Input: part model. Units: mm. Frame: model coordinates. A direction names the side the tool comes from. Coordinates: 2 decimals unless noted, no trailing zeros. Order: outer loops, then holes, each group sorted by start corner. A loop starts at its lowest first (then second) coordinate and runs counter-clockwise, first axis right, second up.
from build123d import *

# Parameters (mm, degrees)
F1_W     = 2334
F1_H     = 613
F2_DEPTH = 29
F4_DEPTH = 871
F3_W     = 45
F3_H     = 463
F3_W_2   = 392
F3_H_2   = 45
F3_W_3   = 525
F7_DEPTH = 95
F3_W_4   = 70
F8_DEPTH = 750
F6_W     = 2184
F6_H     = 553
F6_W_2   = 45
F6_H_2   = 463
F9_DEPTH = 95


with BuildPart() as f2:
    # F1 (on offset) → F2 (new body)
    with BuildSketch(Plane.XY.offset(900)):
        Rectangle(F1_W, F1_H)
    extrude(amount=-F2_DEPTH)

    # F3 (on face) → F4 (join)
    with BuildSketch(Plane(origin=(0, 0, 871), x_dir=(1, 0, 0), z_dir=(0, 0, -1))):
        Polygon((-1022, 256.5), (-1117, 256.5), (-1117, 211.5), (-1072, 211.5), (-1022, 211.5), align=None)
        Polygon((-1072, -251.5), (-1117, -251.5), (-1117, -296.5), (-1022, -296.5), (-1022, -251.5), align=None)
        Polygon((1117, -296.5), (1117, -251.5), (1072, -251.5), (1022, -251.5), (1022, -296.5), align=None)
        Polygon((1117, 256.5), (1022, 256.5), (1022, 211.5), (1072, 211.5), (1117, 211.5), align=None)
        Polygon((35, 256.5), (-35, 256.5), (-35, 211.5), (-22.5, 211.5), (22.5, 211.5), (35, 211.5), align=None)
        Polygon((22.5, -251.5), (-22.5, -251.5), (-35, -251.5), (-35, -296.5), (35, -296.5), (35, -251.5), align=None)
    extrude(amount=F4_DEPTH)

    # F3 (on face) → F7 (join)
    with BuildSketch(Plane(origin=(0, 0, 871), x_dir=(1, 0, 0), z_dir=(0, 0, -1))):
        with Locations((-1094.5, -20)):
            Rectangle(F3_W, F3_H)
        with Locations((-826, 234)):
            Rectangle(F3_W_2, F3_H_2)
        with Locations((-826, -274)):
            Rectangle(F3_W_2, F3_H_2)
        with Locations((-297.5, -274)):
            Rectangle(F3_W_3, F3_H_2)
        with Locations((-297.5, 234)):
            Rectangle(F3_W_3, F3_H_2)
        with Locations((297.5, 234)):
            Rectangle(F3_W_3, F3_H_2)
        with Locations((297.5, -274)):
            Rectangle(F3_W_3, F3_H_2)
        with Locations((826, -274)):
            Rectangle(F3_W_2, F3_H_2)
        with Locations((826, 234)):
            Rectangle(F3_W_2, F3_H_2)
        with Locations((1094.5, -20)):
            Rectangle(F3_W, F3_H)
    extrude(amount=F7_DEPTH)

    # F3 (on face) → F8 (join)
    with BuildSketch(Plane(origin=(0, 0, 871), x_dir=(1, 0, 0), z_dir=(0, 0, -1))):
        with Locations((-595, 234)):
            Rectangle(F3_W_4, F3_H_2)
        with Locations((-595, -274)):
            Rectangle(F3_W_4, F3_H_2)
        with Locations((595, -274)):
            Rectangle(F3_W_4, F3_H_2)
        with Locations((595, 234)):
            Rectangle(F3_W_4, F3_H_2)
    extrude(amount=F8_DEPTH)

    # F6 (on offset) → F9 (join)
    with BuildSketch(Plane.XY.offset(176)):
        with Locations((0, 20)):
            Rectangle(F6_W, F6_H)
        Polygon((-617.5, -211.5), (-1047, -211.5), (-1047, 251.5), (-617.5, 251.5), (-572.5, 251.5), (-22.5, 251.5), (22.5, 251.5), (572.5, 251.5), (617.5, 251.5), (1047, 251.5), (1047, -211.5), (617.5, -211.5), (572.5, -211.5), (22.5, -211.5), (-22.5, -211.5), (-572.5, -211.5), align=None, mode=Mode.SUBTRACT)
        with Locations((-595, 20)):
            Rectangle(F6_W_2, F6_H_2)
        with Locations((0, 20)):
            Rectangle(F6_W_2, F6_H_2)
        with Locations((595, 20)):
            Rectangle(F6_W_2, F6_H_2)
    extrude(amount=-F9_DEPTH)


solid = f2.part
Item 1: Pin query (flat end, axial travel): pin 1 Ø13.5 at (x, y) = (1074.5, 85) entering from -Z; pin 2 Ø13.5 at (y, z) = (-223.5, 60) entering from -X; pin 3 Ø1 at (x, z) = (28, 203.5) entering from +Y. Return the tip coordinate at first contact, or that it passes through.
Response values:
pin 1: stops at z = 81
pin 2: stops at x = -1117
pin 3: stops at y = 296.5
Item 2: Cut plane B-B on x = 792.5. Return loops of the section in (y, z).
Response values:
outline: (-306.5, 871) - (-256.5, 871) - (-256.5, 776) - (-211.5, 776) - (-211.5, 871) - (251.5, 871) - (251.5, 776) - (296.5, 776) - (296.5, 871) - (306.5, 871) - (306.5, 900) - (-306.5, 900) - close; (-256.5, 81) - (-211.5, 81) - (-211.5, 176) - (-256.5, 176) - close; (251.5, 81) - (296.5, 81) - (296.5, 176) - (251.5, 176) - close
Item 3: Ray query, probe 1 along X at (y, z) = (-227.5, 418.5); probe 2 along X at (y, z) = (241.5, 108.5); probe 3 along Y at (x, z) = (9, 457). Return the intervals inside material, ascending.
Response values:
probe 1: x = -1117 to -1022, -630 to -560, -35 to 35, 560 to 630, 1022 to 1117
probe 2: x = -1092 to -1047, -617.5 to -572.5, -22.5 to 22.5, 572.5 to 617.5, 1047 to 1092
probe 3: y = -256.5 to -211.5, 251.5 to 296.5
Item 4: Draft query along X for faces 5 (the face through (1069, 23, 176)), 6 (the face through (-630, 274, 480)). Return one class per face: pulls with the +X half, pulls with the -X half, needs draft (parallel to the pull), parting line crosses it, or undercut.
Response values:
face 5: needs draft
face 6: undercut
Item 5: Access query for faces 1 (the face through (572.5, 17, 129)), 2 (the face through (1072, 23, 824)), 3 (the face through (35, -234, 41)), 4 (the face through (35, -234, 480)). Directions: +Z, -Z, +X, -X, +Y, -Y. A direction counts if a zero-diameter tool reaches every point of the face in a straight line with its end or side. Return the directions, or none.
Response values:
face 1: -Z
face 2: none
face 3: -Z, +Y, -Y
face 4: +Y, -Y
Item 6: Cut plane A-A on y = -235. Count the separate pieces of the cut face and the enclosed holes in it, then the cut area to 3 significant figures.
Response values:
separate pieces: 1
enclosed holes: 4
area: 753,000 mm2
